Part print with two shaded views. Sizes in mm from the minimum x, y, z corner. A direction names the side the tool comes from. Round coordinates to 2 decimals unless told otherwise and drop trailing zeros. Order: outer loops, then holes, each group sorted by start corner. A loop starts at its lowest first (then second) coordinate and runs counter-clockwise, first axis right, second up. Notation, with made-up numbers: (79.25, -15) - (97.25, -15) arc R20 cw to (97.25, 19) - close; hole circle Ø10 at (42.5, 39). An arc over 180 degrees is marked (long way). Use one line per item in the form item = value.
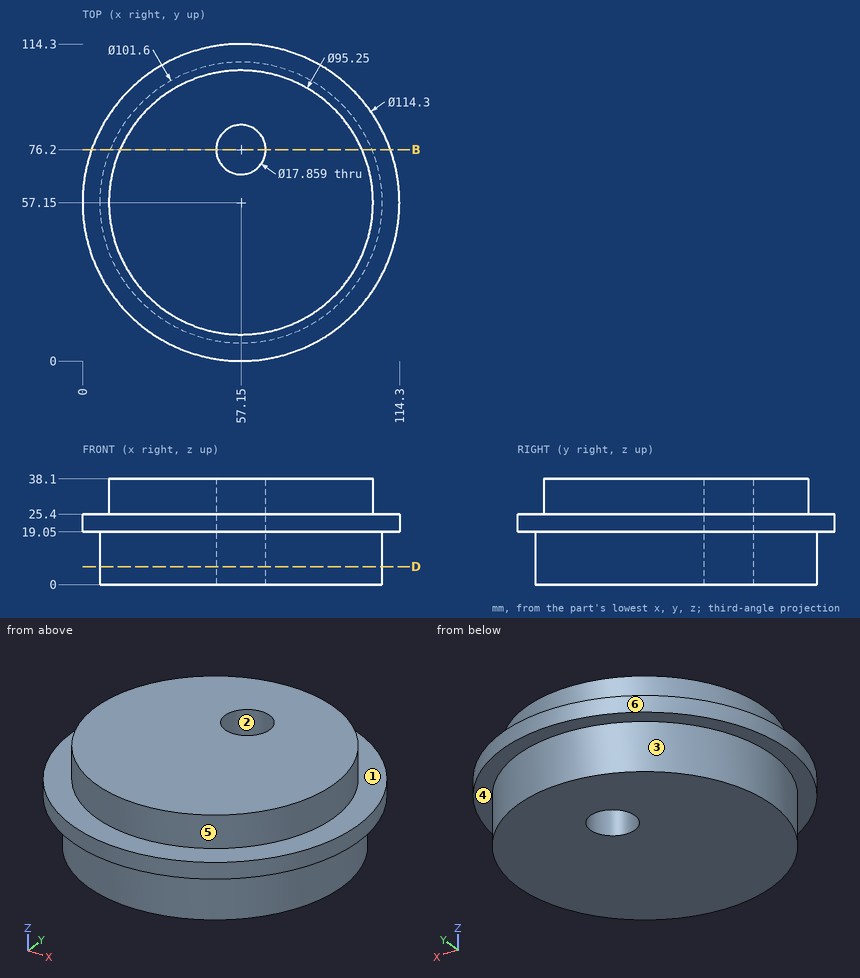
(1) Probe probe 1 along Y at (x, z) = (57.15, 30.5) (1 decimal); probe 2 along Y at (x, z) = (57, 8); probe 3 along Y at (x, z) = (39.5, 17.5) (1 decimal). List the from-to ranges inside material, lowest first. Write a range as [from, to].
Report:
probe_1 = [9.5, 67.3], [85.1, 104.8]
probe_2 = [6.35, 67.27], [85.13, 107.95]
probe_3 = [9.5, 104.8]
(2) Pin check, flat tips, straight feed: pin 1 (12 mm diameter, centred on x = 50, z = 15.5, fed in from +Y); pin 2 (4 mm diameter, centred on x = 76, z = 11.5, fed in from -Y); pin 3 (5 mm diameter, centred on y = 50, z = 6, fed in from +X). Stop position of each tip, or through.
Report:
pin_1 = 114.25
pin_2 = 9.23
pin_3 = 107.74
(3) Slice it at B-B on y = 76.2. Give the cut face in (x, z), then the cut area to 3 significant figures.
Report:
outline = (3.27, 19.05) - (10.06, 19.05) - (10.06, 0) - (48.22, 0) - (48.22, 38.1) - (13.5, 38.1) - (13.5, 25.4) - (3.27, 25.4) - close; (66.08, 0) - (104.24, 0) - (104.24, 19.05) - (111.03, 19.05) - (111.03, 25.4) - (100.8, 25.4) - (100.8, 38.1) - (66.08, 38.1) - close
area = 2,910 mm2
(4) Tool access for the marked faces 4, 5 and 6: list every direction of +Z, -Z, +X, -X, +Y, -Y with a clear straight run to the whole face (end or side of a thin tool).
Report:
face_4 = -Z
face_5 = +Z
face_6 = +Z, -Z
(5) Pull direction X, two halves, no side cores. Call the marked faces 1, 2 and 3: released by +X, released by -X, zero draft, split by the parting line, or undercut.
Report:
face_1 = zero draft
face_2 = undercut
face_3 = split by the parting line
(6) Slice it at D-D on z = 6.5. Give the cut face in (x, y).
Report:
outline = circle Ø101.6 at (57.15, 57.15); hole circle Ø17.86 at (57.15, 76.2)
